Can you work these out from the model? Positions are in its coordinate system, mm. Face numbers are marked on the shaded views. A direction names the side the tool comes from. Round coordinates to 2 decimals unless told otherwise and drop trailing zeros. Loops run counter-clockwise (first coordinate to the right, second up) from the corner with the lowest first, then second, coordinate; pieces in that order, holes last. Notation, with made-up numbers: M 14,80 L 50,80 A17 ccw 50,102 Z; hole C 65.5,70.25 d8. An arc over 180 degrees is marked long. Return JSON: item names as keys, results as strings.
```python
from build123d import *

# Parameters (mm, degrees)
F0_W     = 1200
F0_H     = 300
F1_DEPTH = 700
F2_W     = 600
F2_H     = 100
F3_DEPTH = 700
F4_R     = 160
F5_DEPTH = 700.001
F7_DEPTH = 300.001
F8_W     = 320
F8_H     = 240
F9_DEPTH = 1200.001


with BuildPart() as f1:
    # F0 (on Front) → F1 (new body)
    with BuildSketch(Plane.XZ):
        Rectangle(F0_W, F0_H)
    extrude(amount=F1_DEPTH)

    # F2 (on face) → F3 (join)
    with BuildSketch(Plane(origin=(0, 0, 0), x_dir=(-1, 0, 0), z_dir=(0, 1, 0))):
        with Locations((300, 200)):
            Rectangle(F2_W, F2_H)
        with BuildLine():
            Line((0, 250), (600, 250))
            ThreePointArc((600, 250), (300, 550), (0, 250))
        make_face()
    extrude(amount=-F3_DEPTH)

    # F4 (on face) → F5 (cut, through all)
    with BuildSketch(Plane(origin=(0, 0, 0), x_dir=(-1, 0, 0), z_dir=(0, 1, 0))):
        with Locations((300, 250)):
            Circle(F4_R)
    extrude(amount=-F5_DEPTH, mode=Mode.SUBTRACT)

    # F6 (on face) → F7 (cut, through all)
    with BuildSketch(Plane.XY.offset(150)):
        with BuildLine():
            Line((450, -109.617759), (290, -109.617759))
            ThreePointArc((290, -109.617759), (254.644661, -124.26242), (240, -159.617759))
            Line((240, -159.617759), (240, -519.617759))
            ThreePointArc((240, -519.617759), (254.644661, -554.973098), (290, -569.617759))
            Line((290, -569.617759), (450, -569.617759))
            ThreePointArc((450, -569.617759), (485.355339, -554.973098), (500, -519.617759))
            Line((500, -519.617759), (500, -159.617759))
            ThreePointArc((500, -159.617759), (485.355339, -124.26242), (450, -109.617759))
        make_face()
    extrude(amount=-F7_DEPTH, mode=Mode.SUBTRACT)

    # F8 (on face) → F9 (cut, through all)
    with BuildSketch(Plane.YZ.offset(600)):
        with Locations((-350, -150)):
            Rectangle(F8_W, F8_H)
    extrude(amount=-F9_DEPTH, mode=Mode.SUBTRACT)


solid = f1.part
```
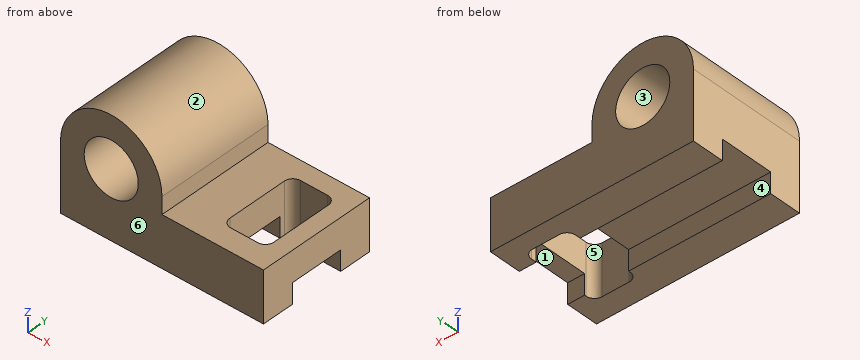
Q1. Suppose I cut it at B-B, the plane x = 334. Please give me the cut outline in (y, z).
Results:
{"outline": "M -700,-150 L -569.62,-150 L -569.62,150 L -700,150 Z; M -109.62,-150 L 0,-150 L 0,150 L -109.62,150 Z"}
Q2. Suppose I cut it at C-C, the plane y = -47.5. Please give me the cut outline in (x, z), plus the area to 3 significant figures.
Results:
{"outline": "M -600,-150 L 600,-150 L 600,150 L 0,150 L 0,250 A300 ccw -600,250 Z; hole C -300,250 d320", "area": "481,000 mm2"}
Q3. Suppose I cut it at D-D, the plane z = 364.5. Please give me the cut outline in (x, y), plus the area to 3 significant figures.
Results:
{"outline": "M -577.29,-700 L -411.76,-700 L -411.76,0 L -577.29,0 Z; M -188.24,-700 L -22.71,-700 L -22.71,0 L -188.24,0 Z", "area": "232,000 mm2"}
Q4. I'm going to push flat-ended pins straight in: pin 1 Ø10 at (y, z) = (-240, 334) entering from +X; pin 2 Ø2 at (y, z) = (-518.5, 200) entering from +X; pin 3 Ø5 at (y, z) = (-343, 348.5) entering from +X. Where does each tip first touch, or does it pass through?
Results:
{"pin 1": "stops at x = -10.59", "pin 2": "stops at x = 0", "pin 3": "stops at x = -15.77"}
Q5. On a 3-axis mill with a long thin cutter (end or side, diameter ignored), from which of +Z, -Z, +X, -X, +Y, -Y can I reach the whole of each face in a straight line? I mean the marked faces 4, 5 and 6. Say none if no direction works.
Results:
{"face 4": "-Z, +X, -X", "face 5": "+Z, -Z", "face 6": "+Z, -Z, +X, -X, -Y"}
Q6. If I drill on line 1 along Z through (x, y) = (-300, -473); line 2 along Y through (x, z) = (68, -58); line 3 along Z through (x, y) = (-296.5, -61.5), over which ranges is the centre line in solid material (lowest first)?
Results:
{"line 1": "z = -30 to 90, 410 to 550", "line 2": "y = -700 to -510, -190 to 0", "line 3": "z = -150 to 90.04, 409.96 to 549.98"}
Q7. Thinking about a two-plate mould opening in X: for the marked faces 1, 2 and 3, which applies, pulls with the +X half, pulls with the -X half, needs draft (parallel to the pull), parting line crosses it, or undercut?
Results:
{"face 1": "needs draft", "face 2": "parting line crosses it", "face 3": "undercut"}
Q8. Suppose I cut it at A-A, the plane y = -404. Please give me the cut outline in (x, z), plus the area to 3 significant figures.
Results:
{"outline": "M -600,-30 L 240,-30 L 240,150 L 0,150 L 0,250 A300 ccw -600,250 Z; M 500,-30 L 600,-30 L 600,150 L 500,150 Z; hole C -300,250 d320", "area": "290,000 mm2"}
